from build123d import *

# Parameters (mm, degrees)
SKETCH1_W           = 106
SKETCH1_H           = 35
BOSS_EXTRUDE1_DEPTH = 26
FILLET1_R           = 2
SKETCH2_R           = 2
BOSS_EXTRUDE2_DEPTH = 10


with BuildPart() as part:
    # Sketch1 → Boss-Extrude1 (new body)
    with BuildSketch(Plane(origin=(0, 0, 0), x_dir=(1, 0, 0), z_dir=(0, 1, 0))):
        Rectangle(SKETCH1_W, SKETCH1_H)
    extrude(amount=BOSS_EXTRUDE1_DEPTH)

    # Fillet1
    fillet1_edges = [part.edges().sort_by_distance(p)[0] for p in [
        (-53, 26, 0),
        (0, 26, 17.5),
        (53, 26, 0),
        (0, 0, 17.5),
        (-53, 0, 0),
        (0, 0, -17.5),
        (53, 0, 0),
        (53, 13, 17.5),
        (-53, 13, 17.5),
        (-53, 13, -17.5),
        (53, 13, -17.5),
        (0, 26, -17.5),
    ]]
    fillet(fillet1_edges, radius=FILLET1_R)

    # Sketch2 → Boss-Extrude2 (add)
    with BuildSketch(Plane(origin=(53, 0, 0), x_dir=(0, 0, -1), z_dir=(1, 0, 0))):
        with Locations((-12.5, 6.5)):
            Circle(SKETCH2_R)
        with Locations((-12.5, 12.5)):
            Circle(SKETCH2_R)
    extrude(amount=BOSS_EXTRUDE2_DEPTH)


solid = part.part
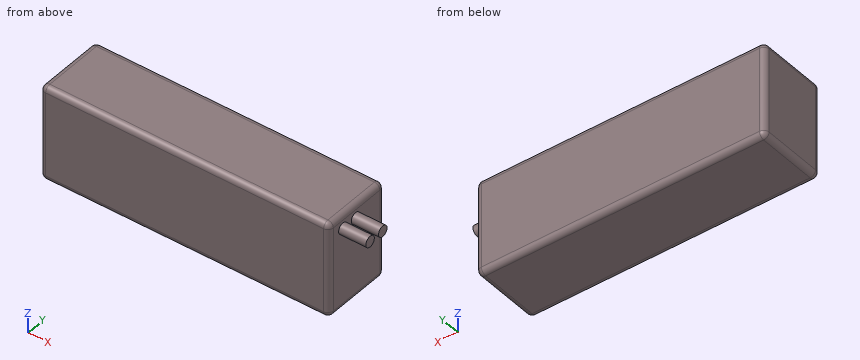
For this review, take the finished solid that the model builds, in its own axes (mm). Coordinates: 2 decimals unless noted, no trailing zeros. Order: outer loops, then holes, each group sorted by start corner. A loop starts at its lowest first (then second) coordinate and runs counter-clockwise, first axis right, second up. Notation, with made-up numbers: (34, -25) - (62, -25) arc R15 ccw to (62, -6) - close; hole circle Ø6 at (79.5, 42). An arc over 180 degrees is marked (long way). Answer as CSV lines item,"result". Start each with the question number.
1) Add section C-C (z = -4). State the section outline as (x, y) points, then the cut area to 3 significant figures.
2) To check wall thickness, follow line 1 along Z through (x, y) = (-23, 1.75); line 2 along X through (y, z) = (24, 5); line 3 along Z through (x, y) = (56, 11). State the ranges of each line that lie inside material, in increasing order. Write a range as [from, to].
3) Insertion check: P1, Ø5, axis at y = 22.5, z = -9, coming from the +X side. The pin has a flat end and moves straight along its axis. Give the tip position at first contact, or say it passes through.
4) Add section A-A (z = 12.5). State the section outline as (x, y) points.
5) Add section B-B (y = 12.5). State the section outline as (x, z) points, then the cut area to 3 significant figures.
Result:
1,outline,"(-53, 2) arc R2 ccw to (-51, 0) - (51, 0) arc R2 ccw to (53, 2) - (53, 24) arc R2 ccw to (51, 26) - (-51, 26) arc R2 ccw to (-53, 24) - close"
1,area,"2,750 mm^2"
2,line 1,"[-17.48, 17.48]"
2,line 2,"[-53, 53]"
2,line 3,"[11.18, 13.82]"
3,P1,"x = 53"
4,outline,"(-53, 2) arc R2 ccw to (-51, 0) - (51, 0) arc R2 ccw to (53, 2) - (53, 4.5) - (63, 4.5) - (63, 8.5) - (53, 8.5) - (53, 10.5) - (63, 10.5) - (63, 14.5) - (53, 14.5) - (53, 24) arc R2 ccw to (51, 26) - (-51, 26) arc R2 ccw to (-53, 24) - close"
5,outline,"(-53, -15.5) arc R2 ccw to (-51, -17.5) - (51, -17.5) arc R2 ccw to (53, -15.5) - (53, 10.5) - (63, 10.5) - (63, 14.5) - (53, 14.5) - (53, 15.5) arc R2 ccw to (51, 17.5) - (-51, 17.5) arc R2 ccw to (-53, 15.5) - close"
5,area,"3,750 mm^2"
